Verification items for this drawing (mm, ordinates from the low corner). Coordinates: 2 decimals unless noted, no trailing zeros. Order: outer loops, then holes, each group sorted by start corner. A loop starts at its lowest first (then second) coordinate and runs counter-clockwise, first axis right, second up.
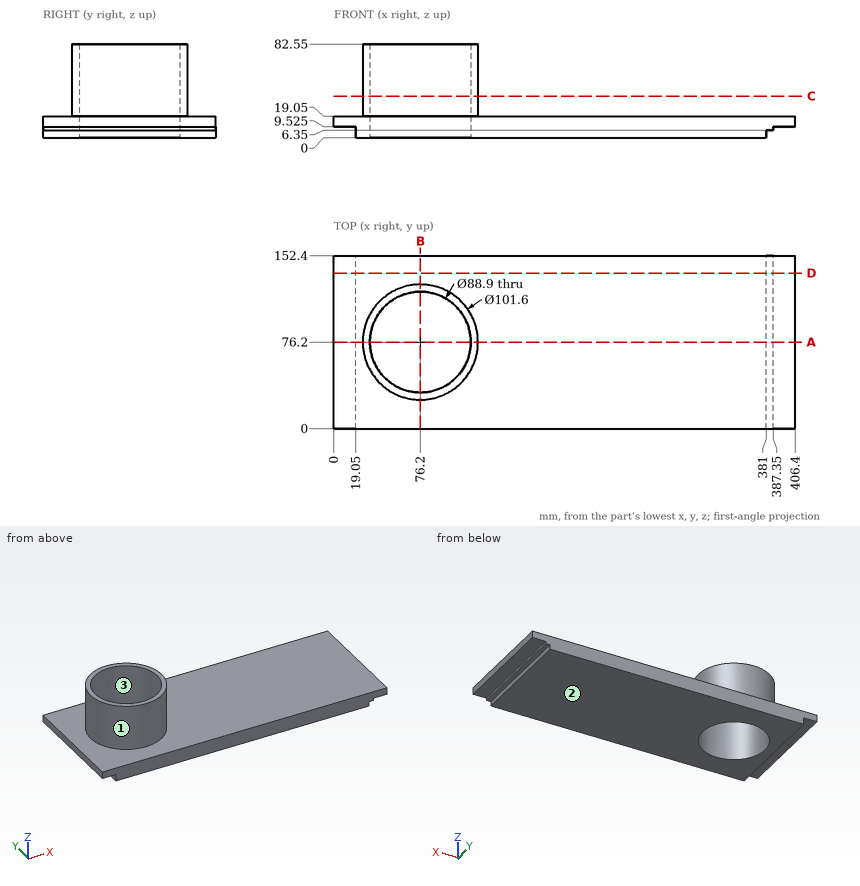
(1) Cross-section at B-B (x = 76.2). Enter the section's corners in (y, z).
Filled in:
outline: (0, 0) - (31.75, 0) - (31.75, 82.55) - (25.4, 82.55) - (25.4, 19.05) - (0, 19.05) - close; (120.65, 0) - (152.4, 0) - (152.4, 19.05) - (127, 19.05) - (127, 82.55) - (120.65, 82.55) - close
(2) Go/stop test with flat-tipped pins: P1, Ø3, axis at x = 304.5, y = 72, coming from the +Z side; P2, Ø1.9, axis at x = 384, y = 47, coming from the -Z side; P3, Ø6, axis at y = 83, z = 55.5, coming from the -X side. Record where each tip stops, or that it passes through.
Filled in:
P1: stops at z = 19.05
P2: stops at z = 6.35
P3: stops at x = 25.54
(3) Cross-section at C-C (z = 36.5). Enter the section's corners in (x, y).
Filled in:
outline: circle Ø101.6 at (76.2, 76.2); hole circle Ø88.9 at (76.2, 76.2)
(4) Cross-section at D-D (y = 137). Enter the section's corners in (x, z) (3 decimals).
Filled in:
outline: (0, 9.525) - (19.05, 9.525) - (19.05, 0) - (381, 0) - (381, 6.35) - (387.35, 6.35) - (387.35, 9.525) - (406.4, 9.525) - (406.4, 19.05) - (0, 19.05) - close
(5) Cross-section at A-A (y = 76.2). Enter the section's corners in (x, z) (3 decimals).
Filled in:
outline: (0, 9.525) - (19.05, 9.525) - (19.05, 0) - (31.75, 0) - (31.75, 82.55) - (25.4, 82.55) - (25.4, 19.05) - (0, 19.05) - close; (120.65, 0) - (381, 0) - (381, 6.35) - (387.35, 6.35) - (387.35, 9.525) - (406.4, 9.525) - (406.4, 19.05) - (127, 19.05) - (127, 82.55) - (120.65, 82.55) - close
(6) Thickness scan on probe 1 along X at (y, z) = (76, 38); probe 2 along Z at (x, y) = (297, 18.5). Record the ranges inside material, lowest first.
Filled in:
probe 1: x = 25.4 to 31.75, 120.65 to 127
probe 2: z = 0 to 19.05
(7) Release check for a two-part mould opening along X. For the marked faces 1, 2 and 3 record: +X half, -X half, draft (parallel to the pull), parting line (faces both ways), or undercut.
Filled in:
face 1: parting line
face 2: draft
face 3: undercut
